The model under review builds one solid part; all positions refer to its coordinate system, in mm. Face numbers are marked on the shaded views. A direction names the side the tool comes from. Round coordinates to 2 decimals unless told otherwise and drop trailing zeros. Write each loop counter-clockwise with the first axis right and the second up, starting at its lowest first coordinate (ties: lowest second). Pieces come first, ordered by that corner, then holes. Notation, with made-up numbers: M 41,76.5 L 100,76.5 A22 cw 100,105.5 Z; hole C 22.5,-22.5 d7. An arc over 180 degrees is marked long. One line per item, written item: value. Start each with the question number.
1) Wall thickness on probe 1 along X at (y, z) = (24, 14.5); probe 2 along X at (y, z) = (11, 15.25); probe 3 along Z at (x, y) = (-9, 6): over which ranges is each line inside the solid? List them lowest first.
2) Take a section at A-A, the plane z = 15. Write out the cut boundary in (x, y), and give its area (3 significant figures).
3) Take a section at C-C, the plane z = 2. Write out the cut boundary in (x, y), and give its area (3 significant figures).
4) Take a section at D-D, the plane x = 9. Write out the cut boundary in (y, z).
5) Tool access review of the marked faces 5, 6, 7, 8 and 9: name each direction out of +Z, -Z, +X, -X, +Y, -Y from which nothing blocks a thin tool from reaching the whole face with its end or side.
6) Mouldability with a two-part tool opening along X and no side actions: class the marked faces 1, 2, 3 and 4 as +X half, -X half, draft (parallel to the pull), parting line (faces both ways), or undercut.
7) Take a section at B-B, the plane y = 15. Write out the cut boundary in (x, z).
8) For P1, Ø2, axis at x = 14.5, y = 13.5, coming from the -Z side; P2, Ø1, axis at x = 12.5, z = 2.5, coming from the +Y side; P3, Ø6.5, axis at y = 5.5, z = 13, coming from the +X side, all flat-tipped, find the tip position at first contact; note any pin that passes through.
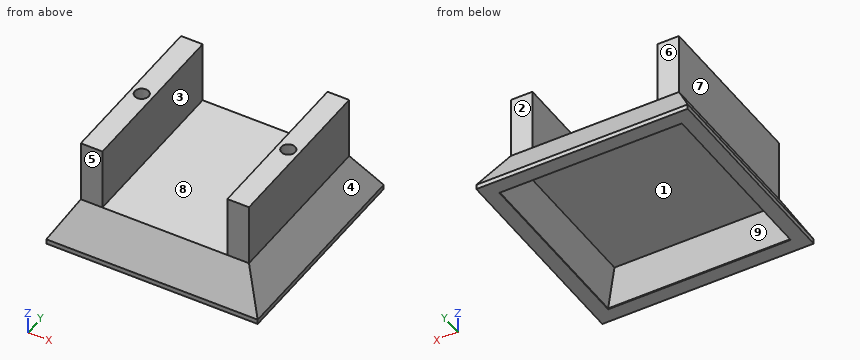
from build123d import *

# Parameters (mm, degrees)
F0_W     = 44
F0_H     = 44
F1_DEPTH = 9
F2_SIZE2 = 8
F2_SIZE  = 4.5
F4_T     = -3
F5_W     = 4.5
F5_H     = 35
F6_DEPTH = 13
F7_R     = 1.45
F8_DEPTH = 13


with BuildPart() as f1:
    # F0 (on Top) → F1 (new body)
    with BuildSketch(Plane.XY):
        with Locations((3.1474529505, 10.1189251319)):
            Rectangle(F0_W, F0_H)
    extrude(amount=F1_DEPTH)

    # F2
    f2_edges = [f1.edges().sort_by_distance(p)[0] for p in [
        (3.147453, -11.881075, 9),
        (-18.852547, 10.118925, 9),
        (3.147453, 32.118925, 9),
        (25.147453, 10.118925, 9),
    ]]
    f2_side = f1.faces().sort_by_distance((3.147453, 10.118925, 9))[0]
    chamfer(f2_edges, length=F2_SIZE, length2=F2_SIZE2, reference=f2_side)

    # F4
    f4_openings = [f1.faces().sort_by_distance(p)[0] for p in [
        (3.147453, 10.118925, 0),
    ]]
    offset(amount=F4_T, openings=f4_openings)

    # F5 (on face) → F6 (join)
    with BuildSketch(Plane.XY.offset(9)):
        with Locations((18.3974529505, 10.1189251319)):
            Rectangle(F5_W, F5_H)
        with Locations((-12.1025470495, 10.1189251319)):
            Rectangle(F5_W, F5_H)
    extrude(amount=F6_DEPTH)

    # F7 (on face) → F8 (cut)
    with BuildSketch(Plane.XY.offset(22)):
        with Locations((-12.1025470495, 10.1189251319)):
            Circle(F7_R)
        with Locations((18.3974529505, 10.1189251319)):
            Circle(F7_R)
    extrude(amount=-F8_DEPTH, mode=Mode.SUBTRACT)


solid = f1.part
Checked values:
1. probe 1: x = -14.35 to -9.85, 16.15 to 20.65
1. probe 2: x = -14.35 to -13.25, -10.95 to -9.85, 16.15 to 17.25, 19.55 to 20.65
1. probe 3: z = 6 to 9
2. outline: M -14.35,-7.38 L -9.85,-7.38 L -9.85,27.62 L -14.35,27.62 Z; M 16.15,-7.38 L 20.65,-7.38 L 20.65,27.62 L 16.15,27.62 Z; hole C -12.1,10.12 d2.9; hole C 18.4,10.12 d2.9
2. area: 302 mm2
3. outline: M -18.29,-11.32 L 24.58,-11.32 L 24.58,31.56 L -18.29,31.56 Z; hole M -14.85,-7.88 L 21.14,-7.88 L 21.14,28.11 L -14.85,28.11 Z
3. area: 543 mm2
4. outline: M -11.88,0 L -8.88,0 L -8.88,0.21 L -5.63,6 L 25.86,6 L 29.12,0.21 L 29.12,0 L 32.12,0 L 32.12,1 L 27.62,9 L -7.38,9 L -11.88,1 Z
5. face 5: +Z, +X, -X, -Y
5. face 6: +Z, +X, -X, +Y
5. face 7: +Z, -X, +Y, -Y
5. face 8: +Z, +Y, -Y
5. face 9: -Z
6. face 1: undercut
6. face 2: draft
6. face 3: undercut
6. face 4: +X half
7. outline: M -18.85,0 L -15.85,0 L -15.85,0.21 L -12.6,6 L 18.89,6 L 22.15,0.21 L 22.15,0 L 25.15,0 L 25.15,1 L 20.65,9 L 20.65,22 L 16.15,22 L 16.15,9 L -9.85,9 L -9.85,22 L -14.35,22 L -14.35,9 L -18.85,1 Z
8. P1: stops at z = 6
8. P2: stops at y = 31.56
8. P3: stops at x = 20.65
